CAD build for the part. Positions are in the model's coordinates, mm. Face numbers are marked on the shaded views. A direction names the side the tool comes from. Give positions to 0.01 mm unless a question says otherwise; leave off trailing zeros. Write each loop counter-clockwise with the first axis right and the second up, starting at its lowest first coordinate (ties: lowest second). Pieces come first, ordered by that corner, then holes. Notation, with made-up numbers: (65.5, 87) - (95.5, 87) arc R30 ccw to (95.5, 121) - close; hole circle Ø9 at (23.25, 38.25). An arc over 180 degrees is marked (long way). Write item = value, one per line. Start each with the question number.
```python
from build123d import *

# Parameters (mm, degrees)
SKETCH1_W           = 38
SKETCH1_H           = 38
SKETCH1_R           = 1
BOSS_EXTRUDE1_DEPTH = 1.3
BOSS_EXTRUDE2_DEPTH = 8.7
SKETCH3_R           = 7
BOSS_EXTRUDE3_DEPTH = 8.6


with BuildPart() as part:
    # Sketch1 → Boss-Extrude1 (new body)
    with BuildSketch(Plane(origin=(0, 0, 0), x_dir=(1, 0, 0), z_dir=(0, 1, 0))):
        with Locations((4.613461538, -5.005769231)):
            Rectangle(SKETCH1_W, SKETCH1_H)
        with Locations(Location((-12.386538462, 11.994230769, 0), (0, 0, 270))):
            Circle(SKETCH1_R, mode=Mode.SUBTRACT)
        with Locations(Location((21.613461538, 11.994230769, 0), (0, 0, 270))):
            Circle(SKETCH1_R, mode=Mode.SUBTRACT)
        with Locations(Location((21.613461538, -22.005769231, 0), (0, 0, 270))):
            Circle(SKETCH1_R, mode=Mode.SUBTRACT)
        with Locations(Location((-12.386538462, -22.005769231, 0), (0, 0, 270))):
            Circle(SKETCH1_R, mode=Mode.SUBTRACT)
    extrude(amount=BOSS_EXTRUDE1_DEPTH)

    # Sketch2 → Boss-Extrude2 (add)
    with BuildSketch(Plane(origin=(0, 1.3, 0), x_dir=(1, 0, 0), z_dir=(0, 1, 0))):
        with BuildLine():
            Line((-1.886538462, -11.505769231), (11.113461538, -11.505769231))
            Line((11.113461538, -11.505769231), (11.113461538, -7.333742244))
            Line((11.113461538, -7.333742244), (13.613461538, -7.333742244))
            ThreePointArc((13.613461538, -7.333742244), (15.941434552, -5.005769231), (13.613461538, -2.677796217))
            Line((13.613461538, -2.677796217), (11.113461538, -2.677796217))
            Line((11.113461538, -2.677796217), (11.113461538, 1.494230769))
            Line((11.113461538, 1.494230769), (-1.886538462, 1.494230769))
            Line((-1.886538462, 1.494230769), (-1.886538462, -2.677796217))
            Line((-1.886538462, -2.677796217), (-4.386538462, -2.677796217))
            ThreePointArc((-4.386538462, -2.677796217), (-6.714511475, -5.005769231), (-4.386538462, -7.333742244))
            Line((-4.386538462, -7.333742244), (-1.886538462, -7.333742244))
            Line((-1.886538462, -7.333742244), (-1.886538462, -11.505769231))
        make_face()
    extrude(amount=BOSS_EXTRUDE2_DEPTH)

    # Sketch3 → Boss-Extrude3 (add)
    with BuildSketch(Plane(origin=(0, 10, 0), x_dir=(1, 0, 0), z_dir=(0, 1, 0))):
        with Locations(Location((4.613461538, -5.005769231, 0), (0, 0, 68.213210702))):
            Circle(SKETCH3_R)
    extrude(amount=BOSS_EXTRUDE3_DEPTH)


solid = part.part
```
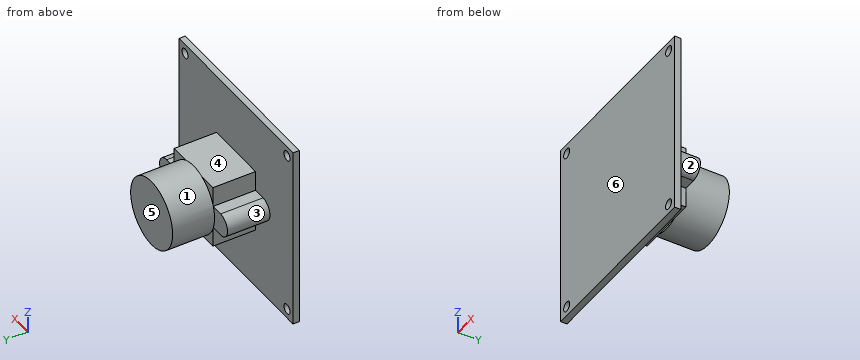
1. Tool access for the marked faces 1 and 2: list every direction of +Z, -Z, +X, -X, +Y, -Y with a clear straight run to the whole face (end or side of a thin tool).
2. Cut at B-B (x = 4). Give the cut face in (y, z).
3. Pin check, flat tips, straight feed: pin 1 Ø3.5 at (y, z) = (4, 10) entering from +X; pin 2 Ø0.8 at (x, y) = (12, 5) entering from -Z; pin 3 Ø3.5 at (y, z) = (5, 8.5) entering from -X; pin 4 Ø10 at (y, z) = (12.5, 19) entering from +X. Stop position of each tip, or through.
4. Cut at D-D (x = 15). Give the cut face in (y, z), then the cut area to 3 significant figures.
5. Mould opens along Y. For the marked faces 3, 4, 5 and 6 say: +Y half, -Y half, draft (parallel to the pull), parting line (faces both ways), or undercut.
6. Cut at C-C (z = -10). Give the cut face in (x, y), then the cut area to 3 significant figures.
7. Wall check: line 1 along Z through (x, y) = (-2, 8.5); line 2 along Y through (x, z) = (-8, 5); line 3 along X through (y, z) = (5.75, 0). Give the ranges that are in metal, low to high.
Output:
q1.face_1 = +Y
q1.face_2 = +X, +Y
q2.outline = (0, -13.99) - (1.3, -13.99) - (1.3, -1.49) - (10, -1.49) - (10, -1.97) - (18.6, -1.97) - (18.6, 11.98) - (10, 11.98) - (10, 11.51) - (1.3, 11.51) - (1.3, 24.01) - (0, 24.01) - close
q3.pin_1 = 11.11
q3.pin_2 = 2.68
q3.pin_3 = -5.93
q3.pin_4 = through
q4.outline = (0, -13.99) - (1.3, -13.99) - (1.3, 3.14) - (10, 3.14) - (10, 6.88) - (1.3, 6.88) - (1.3, 24.01) - (0, 24.01) - close
q4.area = 81.9 mm2
q5.face_3 = draft
q5.face_4 = undercut
q5.face_5 = +Y half
q5.face_6 = -Y half
q6.outline = (-14.39, 0) - (23.61, 0) - (23.61, 1.3) - (-14.39, 1.3) - close
q6.area = 49.4 mm2
q7.line_1 = 2.68 to 7.33
q7.line_2 = 0 to 1.3
q7.line_3 = -1.89 to 11.11
